Verification items for the finished model (mm, model axes). A direction names the side the tool comes from. Give positions to 0.01 mm unless a question says otherwise; leave off trailing zeros. Loops run counter-clockwise (first coordinate to the right, second up) from the corner with the lowest first, then second, coordinate; pieces in that order, holes last. Notation, with made-up numbers: M 59,18 L 81,18 A33 ccw 81,56 Z; hole C 39,58 d2. An arc over 180 degrees is marked long. Use CSV: the item, a comma, the result in double quotes.
from build123d import *

# Parameters (mm, degrees)
SKETCH_W     = 66.5
SKETCH_H     = 70
PAD_DEPTH    = 5
PAD001_DEPTH = 18
PAD002_DEPTH = 5
FILLET_R     = 5
FILLET001_R  = 5
FILLET002_R  = 5
FILLET003_R  = 5
FILLET004_R  = 3
FILLET005_R  = 3
FILLET006_R  = 3


with BuildPart() as part:
    # Sketch → Pad (new body)
    with BuildSketch(Plane.XY):
        Rectangle(SKETCH_W, SKETCH_H)
    extrude(amount=PAD_DEPTH)

    # Sketch001 (on Face6 of Pad) → Pad001 (join)
    with BuildSketch(Plane.XY.offset(5)):
        Polygon((-28.25, -20), (-28.25, 9), (28.25, 9), (28.25, -20), (33.25, -20), (33.25, 14), (-33.25, 14), (-33.25, -20), align=None)
    extrude(amount=PAD001_DEPTH)

    # Sketch002 (on Face11 of Pad001) → Pad002 (join)
    with BuildSketch(Plane.XZ.offset(20)):
        Polygon((-28.25, 23), (-10.25, 5), (-28.25, 5), align=None)
        Polygon((10.25, 5), (28.25, 23), (28.25, 5), align=None)
    extrude(amount=-PAD002_DEPTH)

    # Fillet
    fillet_edges = [part.edges().sort_by_distance(p)[0] for p in [
        (33.25, -35, 2.5),
    ]]
    fillet(fillet_edges, radius=FILLET_R)

    # Fillet001
    fillet001_edges = [part.edges().sort_by_distance(p)[0] for p in [
        (-33.25, -35, 2.5),
    ]]
    fillet(fillet001_edges, radius=FILLET001_R)

    # Fillet002
    fillet002_edges = [part.edges().sort_by_distance(p)[0] for p in [
        (33.25, 35, 2.5),
    ]]
    fillet(fillet002_edges, radius=FILLET002_R)

    # Fillet003
    fillet003_edges = [part.edges().sort_by_distance(p)[0] for p in [
        (-33.25, 35, 2.5),
    ]]
    fillet(fillet003_edges, radius=FILLET003_R)

    # Fillet004
    fillet004_edges = [part.edges().sort_by_distance(p)[0] for p in [
        (33.25, -3, 23),
        (0, 14, 23),
        (-33.25, -3, 23),
    ]]
    fillet(fillet004_edges, radius=FILLET004_R)

    # Fillet005
    fillet005_edges = [part.edges().sort_by_distance(p)[0] for p in [
        (0, 14, 5),
    ]]
    fillet(fillet005_edges, radius=FILLET005_R)

    # Fillet006
    fillet006_edges = [part.edges().sort_by_distance(p)[0] for p in [
        (30.75, -20, 5),
        (-19.25, -20, 5),
        (-30.75, -20, 5),
        (19.25, -20, 5),
    ]]
    fillet(fillet006_edges, radius=FILLET006_R)


solid = part.part
(1) Section check C-C on x = 15.5. Record the cut outline in (y, z), plus the area to 3 significant figures.
Calculated:
outline,"M -35,0 L 35,0 L 35,5 L 17,5 A3 cw 14,8 L 14,20 A3 ccw 11,23 L 9,23 L 9,5 L -15,5 L -15,10.25 L -20,10.25 L -20,8 A3 cw -23,5 L -35,5 Z"
area,"468 mm²"
(2) Section check D-D on y = -24. Record the cut outline in (x, z).
Calculated:
outline,"M -33.25,0 L 33.25,0 L 33.25,5 L -33.25,5 Z"
(3) Section check A-A on z = 16.75. Record the cut outline in (x, y), plus the area to 3 significant figures.
Calculated:
outline,"M -33.25,-20 L -22,-20 L -22,-15 L -28.25,-15 L -28.25,9 L 28.25,9 L 28.25,-15 L 22,-15 L 22,-20 L 33.25,-20 L 33.25,14 L -33.25,14 Z"
area,"685 mm²"
(4) Section check B-B on x = -23. Record the cut outline in (y, z), plus the area to 3 significant figures.
Calculated:
outline,"M -35,0 L 35,0 L 35,5 L 17,5 A3 cw 14,8 L 14,20 A3 ccw 11,23 L 9,23 L 9,5 L -15,5 L -15,17.75 L -20,17.75 L -20,8 A3 cw -23,5 L -35,5 Z"
area,"506 mm²"
(5) Tool access check on faces 4 (the cylindrical face through (31.82, -33.5, 2.54)), 5 (the flat face through (0, 9, 14)), 6 (the flat face through (0, 26, 5)), 7 (the flat face through (19.12, -18.17, 13.87)), 8 (the flat face through (25, -20, 14)). Record the directions out of +Z, -Z, +X, -X, +Y, -Y that give a thin tool (end or side, any length) a straight path to the whole face; none if there is none.
Calculated:
face 4,"+Z, -Z, +X, -Y"
face 5,"+Z"
face 6,"+Z, +X, -X, +Y"
face 7,"+Z, -Y"
face 8,"+Z, +X, -X, -Y"
(6) Mould release check, pull along Y, two halves, no side actions. Record for faces 1 (the flat face through (-25, -20, 14)), 2 (the flat face through (-23, -15, 10)), 3 (the cylindrical face through (-31.75, 33.57, 2.54)): released by +Y, released by -Y, zero draft, split by the parting line, or undercut.
Calculated:
face 1,"released by -Y"
face 2,"undercut"
face 3,"released by +Y"
(7) Depth check by flat-ended pin: pin 1 Ø10 at (y, z) = (-21.5, 7.5) entering from -X; pin 2 Ø12 at (x, z) = (26, 17.5) entering from +Y; pin 3 Ø9 at (x, y) = (-8, 28.5) entering from +Z; pin 4 Ø8 at (x, z) = (-6.5, 10.5) entering from +Y. Enter the tip coordinate at first touch or a pass-through.
Calculated:
pin 1,"stops at x = -33.25"
pin 2,"stops at y = 14"
pin 3,"stops at z = 5"
pin 4,"stops at y = 14.4"
(8) Scan lines: L1, parallel to X at y = -6.5, z = 8.75; L2, parallel to Z at x = -2, y = -19; L3, parallel to Y at x = 27.5, z = 16.75. Record each from-to range of solid material in increasing order. Write a range as from..to.
Calculated:
L1,"x = -33.25..-28.25, 28.25..33.25"
L2,"z = 0..5"
L3,"y = -20..-15, 9..14"
